from build123d import *

# Parameters (mm, degrees)
SKETCH_1_R      = 1.5
EXTRUDE_1_DEPTH = 30


with BuildPart() as part:
    # 草图1 → 凸台-拉伸1 (new body)
    with BuildSketch(Plane.XY):
        Polygon((2.696225757, 0), (1.348112879, 2.335), (-1.348112879, 2.335), (-2.696225757, 0), (-1.348112879, -2.335), (1.348112879, -2.335), align=None)
        Circle(SKETCH_1_R, mode=Mode.SUBTRACT)
    extrude(amount=EXTRUDE_1_DEPTH)

    # 切除-扫描1: sweep along a curve in space
    with BuildLine() as sweep_1_path:
        ThreePointArc((1.5, 0, 0), (1.060660172, 1.060660172, 0), (0, 1.5, 0))
        ThreePointArc((0, 1.5, 0), (-1.060660172, 1.060660172, 0), (-1.5, 0, 0))
        ThreePointArc((-1.5, 0, 0), (-1.060660172, -1.060660172, 0), (0, -1.5, 0))
        ThreePointArc((0, -1.5, 0), (1.060660172, -1.060660172, 0), (1.5, 0, 0))
    # 草图2 → 切除-扫描1 (sweep, cut)
    with BuildSketch(Plane(origin=(0, 0, 0), x_dir=(0, 0, -1), z_dir=(1, 0, 0))):
        Polygon((-0.27716486, 1.42283514), (0.101677918, 1.801677918), (0.101677918, 1.42283514), align=None)
        Polygon((0.0715027, 2.1284973), (-0.9284973, 3.1284973), (0.0715027, 3.1284973), align=None)
        Polygon((-29.72283514, 1.42283514), (-30.101677918, 1.801677918), (-30.101677918, 1.42283514), align=None)
        Polygon((-29.0715027, 3.1284973), (-30.0715027, 3.1284973), (-30.0715027, 2.1284973), align=None)
    sweep(path=sweep_1_path.line, mode=Mode.SUBTRACT)


solid = part.part
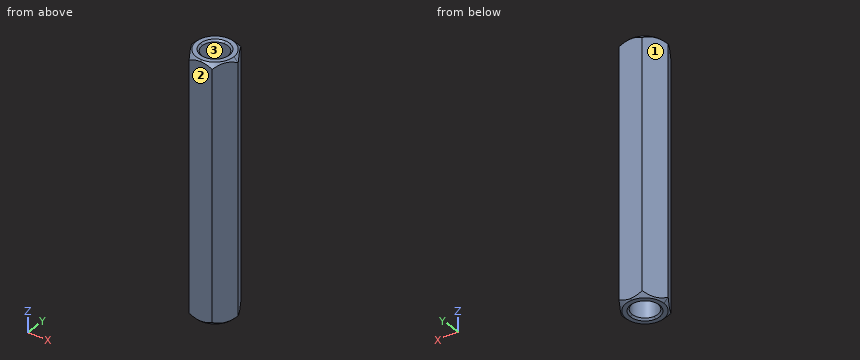
CAD build for the part. Positions are in the model's coordinates, mm. Face numbers are marked on the shaded views. Round coordinates to 2 decimals unless told otherwise and drop trailing zeros. Loops run counter-clockwise (first coordinate to the right, second up) from the corner with the lowest first, then second, coordinate; pieces in that order, holes last.
(1) Two-plate mould, pull along Y, no slides. Class the marked faces 1, 2 and 3: +Y half, -Y half, draft (parallel to the pull), parting line (faces both ways), or undercut.
(2) Wall check: line 1 along Y through (x, z) = (0, 8.75) (3 decimals); line 2 along Y through (x, z) = (0.65, 23.5) (3 decimals); line 3 along X through (y, z) = (0.15, 27). Give the ranges that are in metal, low to high.
(3) Cut at A-A (z = 14). Give the cut face in (x, y) (3 decimals), plus the area to 3 significant figures.
Findings below:
1. face 1: +Y half
1. face 2: -Y half
1. face 3: undercut
2. line 1: y = -2.335 to -1.5, 1.5 to 2.335
2. line 2: y = -2.335 to -1.352, 1.352 to 2.335
2. line 3: x = -2.61 to -1.49, 1.49 to 2.61
3. outline: (-2.696, 0) - (-1.348, -2.335) - (1.348, -2.335) - (2.696, 0) - (1.348, 2.335) - (-1.348, 2.335) - close; hole circle Ø3 at (0, 0)
3. area: 11.8 mm2
